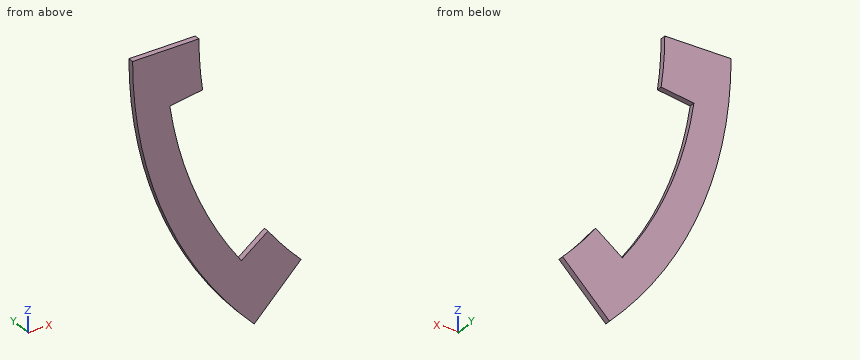
Autodesk Inventor part; units mm, degrees
ref_plane "YZ Plane" through (0, 0, 0) normal (1, 0, 0) x (0, 1, 0)
ref_plane "XZ Plane" through (0, 0, 0) normal (0, 1, 0) x (-1, 0, 0)
ref_plane "XY Plane" through (0, 0, 0) normal (0, 0, 1) x (1, 0, 0)
sketch "スケッチ1" plane through (0, 0, 0) normal (0, 1, 0) x (-1, 0, 0)
  circle A0 centre (0, 0) radius 178.1675
  circle A1 centre (0, 0) radius 157.8276
  line L0 (168.1877, 0) -> (166.7488, -21.9529)
  line L1 (168.1877, 0) -> (130.1721, 2.4917) construction
  line L2 (249.4344, 0) -> (-249.4344, 0)
  line L3 (166.7488, -21.9529) -> (156.7702, -21.2989)
  line L4 (156.7702, -21.2989) -> (158.2091, 0.654) construction
  line L5 (158.2091, 0.654) -> (168.1877, 0)
  line L6 (157.4896, -10.3224) -> (0, 0)
  line L7 (166.7488, -21.9529) -> (162.4568, -43.5302)
  line L8 (162.4568, -43.5302) -> (152.649, -41.5793) construction
  line L9 (152.649, -41.5793) -> (156.9409, -20.002) construction
  line L10 (156.9409, -20.002) -> (166.7488, -21.9529) construction
  line L11 (162.4568, -43.5302) -> (155.3851, -64.3626)
  line L12 (155.3851, -64.3626) -> (145.9158, -61.1482) construction
  line L13 (145.9158, -61.1482) -> (152.9875, -40.3158) construction
  line L14 (152.9875, -40.3158) -> (162.4568, -43.5302) construction
  line L15 (155.3851, -64.3626) -> (145.6548, -84.0938)
  line L16 (145.6548, -84.0938) -> (136.6861, -79.6709) construction
  line L17 (136.6861, -79.6709) -> (146.4164, -59.9397) construction
  line L18 (146.4164, -59.9397) -> (155.3851, -64.3626) construction
  line L19 (0, 0) -> (111.6009, -111.6009)
  line L20 (145.6548, -84.0938) -> (137.3401, -78.5381) construction
  line L21 (137.3401, -78.5381) -> (125.1176, -96.8305) construction
  line L22 (125.1176, -96.8305) -> (133.4323, -102.3862) construction
  line L23 (133.4323, -102.3862) -> (145.6548, -84.0938)
  line L24 (133.4323, -102.3862) -> (125.9139, -95.7927) construction
  line L25 (125.9139, -95.7927) -> (111.4082, -112.3332) construction
  line L26 (111.4082, -112.3332) -> (118.9266, -118.9266)
  line L27 (118.9266, -118.9266) -> (133.4323, -102.3862)
  line L28 (111.6009, -111.6009) -> (118.9266, -118.9266)
  line L29 (166.7488, -21.9529) -> (176.7274, -22.6069) construction
  line L30 (118.9266, -118.9266) -> (125.9834, -125.9834)
  point P0 (154.795, -30.7906)
  point P1 (149.4517, -50.732)
  point P2 (141.5512, -69.8053)
  point P3 (131.2288, -87.6843)
  point P4 (118.661, -104.0629)
  point P5 (157.8276, 0)
  point P6 (178.1675, 0)
  dimension "d0" = 22
  dimension "d1" = 10
  dimension "d2" = 45
  dimension "d4" = 315.6551
extrude "押し出し1" add sketch "スケッチ1" along normal blind 2.5 contours L30 L27 L23 L15 L11 L7 L0 L2 A0 | L28 A1 L2 L0 L7 L11 L15 L23 L27
sketch "スケッチ2" plane through (0, 2.5, 0) normal (0, 1, 0) x (1, 0, 0)
  circle A0 centre (0, 0) radius 277.8276
  line L0 (-168.1877, 0) -> (-166.7488, 21.9529)
  line L1 (-166.7488, 21.9529) -> (-162.4568, 43.5302)
  line L2 (-162.4568, 43.5302) -> (-155.3851, 64.3626)
  line L3 (-155.3851, 64.3626) -> (-145.6548, 84.0938)
  line L4 (-133.4323, 102.3862) -> (-145.6548, 84.0938)
  line L5 (-118.9266, 118.9266) -> (-133.4323, 102.3862)
  line L6 (-167.4682, 10.9764) -> (-166.0294, 32.9293)
  line L7 (-166.0294, 32.9293) -> (-275.7938, 40.1237)
  line L8 (-275.7938, 40.1237) -> (-277.2327, 18.1708)
  line L9 (-277.2327, 18.1708) -> (-167.4682, 10.9764)
  line L10 (-164.6028, 32.7415) -> (-160.3108, 54.3188)
  line L11 (-160.3108, 54.3188) -> (-268.1972, 75.7787)
  line L12 (-268.1972, 75.7787) -> (-272.4892, 54.2015)
  line L13 (-272.4892, 54.2015) -> (-164.6028, 32.7415)
  circle A1 centre (-166.7488, 21.9529) radius 11
  circle A2 centre (-162.4568, 43.5302) radius 11
  line L14 (-158.921, 53.9464) -> (-151.8493, 74.7789)
  line L15 (-151.8493, 74.7789) -> (-256.0116, 110.1372)
  line L16 (-256.0116, 110.1372) -> (-263.0833, 89.3047)
  line L17 (-263.0833, 89.3047) -> (-158.921, 53.9464)
  circle A3 centre (-155.3851, 64.3626) radius 11
  arc A4 (-275.7591, 62.4834) -> (-281.3553, 41.7349) centre (-166.7488, 21.9529) ccw
  line L18 (-178.1663, 0.654) -> (-158.2091, -0.654)
  line L19 (-158.2091, -0.654) -> (-156.7702, 21.2989)
  line L20 (-156.7702, 21.2989) -> (-176.7274, 22.6069)
  line L21 (-176.7274, 22.6069) -> (-178.1663, 0.654)
  line L22 (-177.4468, 11.6305) -> (-275.7938, 40.1237)
  line L23 (-176.7274, 22.6069) -> (-176.008, 33.5834)
  line L24 (-176.008, 33.5834) -> (-275.7591, 62.4834)
  line L25 (-275.7938, 40.1237) -> (-281.3553, 41.7349)
  circle A5 centre (0, 0) radius 137.8276
  line L26 (0, 0) -> (-196.4538, 196.4538)
  line L27 (-111.6009, 111.6009) -> (-125.9834, 125.9834)
  line L28 (-411.1762, 0) -> (411.1762, 0)
  circle A6 centre (0, 0) radius 257.8276 construction
  arc A7 (-111.6009, 111.6009) -> (-157.8276, 0) centre (0, 0) ccw
  point P0 (-158.1662, 0)
  point P1 (-137.8276, 0)
  point P2 (-97.4588, 97.4588)
  point P3 (-277.8276, 0)
  dimension "d7" = 22
  dimension "d10" = 20
  dimension "d11" = 100
  dimension "d12" = 20
  dimension "d14" = 20
  dimension "d17" = 100
extrude "押し出し2" add sketch "スケッチ2" against normal blind 2.5 contours L26 L5 L4 L3 A3 L15 A0 | A0 L9 L21 L18 L28 | L15 A3 L17 A0 | A0 L22 L9 | L18 L21 L9 L0 | L0 A1 L19 L28 | A5 L28 A7 A1 A2 A3 L26 | L17 A2 L11 A0 | A3 L3 L14 | L14 L2 A3 | L26 A7 A3 L3 L4 L5 | A0 L7 L23 A1 L21 L22 | L21 A1 L9 | A1 L21 L20 L0 | L0 L20 L19 A1 | L19 A7 L28 | L11 A2 L13 L24 A0 | A2 A7 L1 L2 | L2 L10 A2 | A3 A7 A2 | L2 L3 A3 A7 | A0 L13 L24 L7 | A1 L23 L21 | L6 A1 L1 | L20 L23 A1 L6 | L1 A1 A7 L19 L20 | A1 A7 L19 | A3 A7 | L24 L13 A0 | L10 L1 A2 | A2 A7 | L24 L13 A1 L7 | L7 A1 L23 | A2 A7 A1 | A7 A1
sketch "スケッチ4" plane through (0, 2.5, 0) normal (0, 1, 0) x (1, 0, 0)
  circle A0 centre (0, 0) radius 187.8276
  arc A1 (-97.4588, 97.4588) -> (-137.8276, 0) centre (0, 0) ccw
  line L0 (-137.5954, 7.9966) -> (-137.8276, 0)
  arc A2 (-196.4538, 196.4538) -> (-277.8276, 0) centre (0, 0) ccw
  line L1 (-97.4588, 97.4588) -> (-196.4538, 196.4538)
  circle A3 centre (0, 0) radius 157.8276
  circle A4 centre (0, 0) radius 172.8276
  line L2 (-97.4588, 97.4588) -> (-196.4538, 196.4538)
  arc A5 (-196.4538, 196.4538) -> (-277.8276, 0) centre (0, 0) ccw
  line L3 (-277.8276, 0) -> (-137.8276, 0)
  arc A6 (-97.4588, 97.4588) -> (-137.8276, 0) centre (0, 0) ccw
  point P0 (-277.3596, 16.1193)
  point P1 (-111.6009, 111.6009)
  point P2 (-157.8276, 0)
  point P3 (-187.8276, 0)
  point P4 (-132.8141, 132.8141)
  point P5 (-277.8276, 0)
  point P6 (-172.8276, 0)
  point P7 (-122.2075, 122.2075)
  dimension "d23" = 50
  dimension "d29" = 20
  dimension "d30" = 15
extrude "押し出し4" cut sketch "スケッチ4" against normal through all contours A0 L3 A4 L1 | A0 L3 A2 L1 | A4 L3 A3 L1 | L1 A3 L3 A4 | A3 L3 L0 A1 L1 | L1 A1 L3 A3 picked at (-124.5192, 133.5739)
sketch "スケッチ5" plane through (0, 2.5, 0) normal (0, 1, 0) x (1, 0, 0)
  line L0 (-136.3765, 19.9473) -> (-185.8501, 27.1836)
  line L1 (-277.8276, 0) -> (-137.8276, 0)
  line L2 (-136.3765, 19.9473) -> (-185.8501, 27.1836)
  arc A0 (-185.8501, 27.1836) -> (-186.1918, 24.735) centre (0, 0) ccw
  arc A1 (-201.9314, 11.7356) -> (-186.1918, 24.735) centre (-201.0611, 26.7104) ccw
  line L3 (-201.9314, 11.7356) -> (-277.3596, 16.1193)
  arc A2 (-277.3596, 16.1193) -> (-277.8276, 0) centre (0, 0) ccw
  line L4 (-277.8276, 0) -> (-137.8276, 0)
  arc A3 (-136.3765, 19.9473) -> (-137.8276, 0) centre (0, 0) ccw
  line L5 (-150.6376, 112.1941) -> (-110.5376, 82.3279)
  arc A4 (-97.4588, 97.4588) -> (-110.5376, 82.3279) centre (0, 0) ccw
  line L6 (-97.4588, 97.4588) -> (-196.4538, 196.4538)
  arc A5 (-196.4538, 196.4538) -> (-207.5209, 184.7248) centre (0, 0) ccw
  line L7 (-207.5209, 184.7248) -> (-151.0854, 134.4887)
  arc A6 (-149.1478, 114.1672) -> (-151.0854, 134.4887) centre (-161.0588, 123.2846) ccw
  arc A7 (-149.1478, 114.1672) -> (-150.6376, 112.1941) centre (0, 0) ccw
  arc A8 (-111.6009, 111.6009) -> (-157.8276, 0) centre (0, 0) ccw
  arc A9 (-122.2075, 122.2075) -> (-172.8276, 0) centre (0, 0) ccw
  point P0 (-171.008, 25.0127)
  point P1 (-156.1659, 22.8418)
  point P2 (-138.6076, 103.2343)
  point P3 (-126.5776, 94.2744)
extrude "押し出し5" add sketch "スケッチ5" against normal up to surface (2.5 mm away) contours A8 L1 A9 L0 | L5 A9 L6 A8
properties part number "belt_rail" material "木材 (カエデ材)"
Verification items for the finished model (mm, model axes). Coordinates: 2 decimals unless noted, no trailing zeros. Order: outer loops, then holes, each group sorted by start corner. A loop starts at its lowest first (then second) coordinate and runs counter-clockwise, first axis right, second up. Notation, with made-up numbers: M 7.25,-1.75 L 35.25,-1.75 A7 ccw 35.25,2.25 Z; hole C 81,16.5 d5. An arc over 180 degrees is marked long. Return JSON: item names as keys, results as strings.
1) Cross-section at C-C, the plane z = -72. Record the boundary of the cut face in (x, y).
Answer list:
{"outline": "M -173.48,0 L -157.12,0 L -157.12,2.5 L -173.48,2.5 Z"}
2) Cross-section at A-A, the plane y = 2.05. Record the boundary of the cut face in (x, z), and give its area (3 significant figures).
Answer list:
{"outline": "M -187.83,0 A187.83 ccw -132.81,-132.81 L -111.6,-111.6 A157.83 cw -126.58,-94.27 L -138.61,-103.23 A172.83 cw -171.01,-25.01 L -156.17,-22.84 A157.83 cw -157.83,0 Z", "area": "2,840 mm2"}
3) Cross-section at B-B, the plane x = -164. Record the boundary of the cut face in (y, z), and give its area (3 significant figures).
Answer list:
{"outline": "M 0,-91.56 L 2.5,-91.56 L 2.5,-54.53 L 0,-54.53 Z; M 0,-23.99 L 2.5,-23.99 L 2.5,0 L 0,0 Z", "area": "153 mm2"}
4) Gauge pin test, flat ends, axial feed: pin 1 (12 mm diameter, centred on x = -156, z = -106.5, fed in from -Y); pin 2 (1.5 mm diameter, centred on x = -132, y = 1, fed in from -Z). Record the tip position at first contact, or that the pin passes through.
Answer list:
{"pin 1": "y = 0", "pin 2": "z = -132.75"}
5) Thickness scan on L1, parallel to Z at x = -158.5, y = 0.95; L2, parallel to Z at x = -160, y = 0.95; L3, parallel to Z at x = -135.5, y = 2.1. Record the ranges inside material, lowest first. Write a range as [from, to].
Answer list:
{"L1": "[-100.78, -68.9], [-23.18, 0]", "L2": "[-98.38, -65.34], [-23.4, 0]", "L3": "[-130.07, -100.92]"}
6) Cross-section at D-D, the plane x = -147.5. Record the boundary of the cut face in (y, z), and give its area (3 significant figures).
Answer list:
{"outline": "M 0,-116.29 L 2.5,-116.29 L 2.5,-90.07 L 0,-90.07 Z", "area": "65.5 mm2"}
